from build123d import *

# Parameters (mm, degrees)
SKETCH1_R           = 4
SKETCH1_R_2         = 11
BOSS_EXTRUDE1_DEPTH = 10
BOSS_EXTRUDE2_DEPTH = 20
BOSS_EXTRUDE3_DEPTH = 5
SKETCH6_R           = 11
CUT_EXTRUDE2_DEPTH  = 7
CUT_EXTRUDE3_REACH  = 123.903
SKETCH3_R           = 4
FILLET1_R           = 5


with BuildPart() as part:
    # Sketch1 → Boss-Extrude1 (new body)
    # profile 1 of 4: a face of its own
    with BuildSketch(Plane(origin=(0, 0, 0), x_dir=(1, 0, 0), z_dir=(0, 1, 0))):
        with BuildLine():
            ThreePointArc((-15.53030303, -17.49196326), (-18.965809959, -17.990656132), (-22.023809524, -19.633836312))
            ThreePointArc((-22.023809524, -19.633836312), (-40.737950416, -24.78942672), (-57.5, -15))
            Line((-57.5, -15), (-57.5, 15))
            ThreePointArc((-57.5, 15), (-40.737950416, 24.78942672), (-22.023809524, 19.633836312))
            ThreePointArc((-22.023809524, 19.633836312), (-18.965809959, 17.990656132), (-15.53030303, 17.49196326))
            ThreePointArc((-15.53030303, 17.49196326), (-10.248929974, 16.842723462), (-5.406818182, 14.63628582))
            ThreePointArc((-5.406818182, 14.63628582), (-2.801045952, 13.422385369), (0.042391304, 12.999930884))
            ThreePointArc((0.042391304, 12.999930884), (13, 0), (0.042391304, -12.999930884))
            ThreePointArc((0.042391304, -12.999930884), (-2.801045952, -13.422385369), (-5.406818182, -14.63628582))
            ThreePointArc((-5.406818182, -14.63628582), (-10.248929974, -16.842723462), (-15.53030303, -17.49196326))
        make_face()
        with Locations((-37.5, 0)):
            Circle(SKETCH1_R, mode=Mode.SUBTRACT)
        Circle(SKETCH1_R_2, mode=Mode.SUBTRACT)
        with Locations((-15, 0)):
            Circle(SKETCH1_R, mode=Mode.SUBTRACT)
    # profile 2 of 4: a face of its own
    with BuildSketch(Plane(origin=(0, 0, 0), x_dir=(1, 0, 0), z_dir=(0, 1, 0))):
        with Locations((-37.5, 0)):
            Circle(SKETCH1_R)
    # profile 3 of 4: a face of its own
    with BuildSketch(Plane(origin=(0, 0, 0), x_dir=(1, 0, 0), z_dir=(0, 1, 0))):
        with Locations((-15, 0)):
            Circle(SKETCH1_R)
    # profile 4 of 4: a face of its own
    with BuildSketch(Plane(origin=(0, 0, 0), x_dir=(1, 0, 0), z_dir=(0, 1, 0))):
        Circle(SKETCH1_R_2)
    extrude(amount=BOSS_EXTRUDE1_DEPTH)

    # Sketch1<3> → Boss-Extrude2 (add)
    with BuildSketch(Plane(origin=(0, 0, 0), x_dir=(1, 0, 0), z_dir=(0, 1, 0))):
        with BuildLine():
            Line((-67.5, -18.027756377), (-67.5, 18.027756377))
            ThreePointArc((-67.5, 18.027756377), (-43.803347329, 34.427718665), (-15.833333333, 27.487370837))
            ThreePointArc((-15.833333333, 27.487370837), (-7.534032816, 26.467136868), (0.075, 22.999877717))
            ThreePointArc((0.075, 22.999877717), (23, 0), (0.075, -22.999877717))
            ThreePointArc((0.075, -22.999877717), (-7.534032816, -26.467136868), (-15.833333333, -27.487370837))
            ThreePointArc((-15.833333333, -27.487370837), (-43.803347329, -34.427718665), (-67.5, -18.027756377))
        make_face()
        with BuildLine():
            Line((-57.5, -15), (-57.5, 15))
            ThreePointArc((-57.5, 15), (-40.737950416, 24.78942672), (-22.023809524, 19.633836312))
            ThreePointArc((-22.023809524, 19.633836312), (-18.965809959, 17.990656132), (-15.53030303, 17.49196326))
            ThreePointArc((-15.53030303, 17.49196326), (-10.248929974, 16.842723462), (-5.406818182, 14.63628582))
            ThreePointArc((-5.406818182, 14.63628582), (-2.801045952, 13.422385369), (0.042391304, 12.999930884))
            ThreePointArc((0.042391304, 12.999930884), (13, 0), (0.042391304, -12.999930884))
            ThreePointArc((0.042391304, -12.999930884), (-2.801045952, -13.422385369), (-5.406818182, -14.63628582))
            ThreePointArc((-5.406818182, -14.63628582), (-10.248929974, -16.842723462), (-15.53030303, -17.49196326))
            ThreePointArc((-15.53030303, -17.49196326), (-18.965809959, -17.990656132), (-22.023809524, -19.633836312))
            ThreePointArc((-22.023809524, -19.633836312), (-40.737950416, -24.78942672), (-57.5, -15))
        make_face(mode=Mode.SUBTRACT)
    extrude(amount=BOSS_EXTRUDE2_DEPTH)

    # Sketch2 → Boss-Extrude3 (add)
    with BuildSketch(Plane(origin=(0, 20, 0), x_dir=(1, 0, 0), z_dir=(0, 1, 0))):
        with BuildLine():
            Line((-77.5, -20.615528128), (-77.5, 20.615528128))
            ThreePointArc((-77.5, 20.615528128), (-48.761384661, 43.568121551), (-12.5, 37.416573868))
            ThreePointArc((-12.5, 37.416573868), (-4.462855904, 35.989145507), (3.075, 32.856420605))
            ThreePointArc((3.075, 32.856420605), (33, 0), (3.075, -32.856420605))
            ThreePointArc((3.075, -32.856420605), (-4.462855904, -35.989145507), (-12.5, -37.416573868))
            ThreePointArc((-12.5, -37.416573868), (-48.761384661, -43.568121551), (-77.5, -20.615528128))
        make_face()
        with BuildLine():
            Line((-57.5, -15), (-57.5, 15))
            ThreePointArc((-57.5, 15), (-40.737950416, 24.78942672), (-22.023809524, 19.633836312))
            ThreePointArc((-22.023809524, 19.633836312), (-18.965809959, 17.990656132), (-15.53030303, 17.49196326))
            ThreePointArc((-15.53030303, 17.49196326), (-10.248929974, 16.842723462), (-5.406818182, 14.63628582))
            ThreePointArc((-5.406818182, 14.63628582), (-2.801045952, 13.422385369), (0.042391304, 12.999930884))
            ThreePointArc((0.042391304, 12.999930884), (13, 0), (0.042391304, -12.999930884))
            ThreePointArc((0.042391304, -12.999930884), (-2.801045952, -13.422385369), (-5.406818182, -14.63628582))
            ThreePointArc((-5.406818182, -14.63628582), (-10.248929974, -16.842723462), (-15.53030303, -17.49196326))
            ThreePointArc((-15.53030303, -17.49196326), (-18.965809959, -17.990656132), (-22.023809524, -19.633836312))
            ThreePointArc((-22.023809524, -19.633836312), (-40.737950416, -24.78942672), (-57.5, -15))
        make_face(mode=Mode.SUBTRACT)
    extrude(amount=BOSS_EXTRUDE3_DEPTH)

    # Sketch6 → Cut-Extrude2 (cut)
    with BuildSketch(Plane(origin=(-57.5, 0, 0), x_dir=(0, 0, -1), z_dir=(1, 0, 0))):
        with Locations((0.437281594, 25)):
            Circle(SKETCH6_R)
    extrude(amount=-CUT_EXTRUDE2_DEPTH, mode=Mode.SUBTRACT)

    # Sketch3 → Cut-Extrude3 (cut, up to next)
    with BuildSketch(Plane.ZY.offset(77.5), mode=Mode.PRIVATE) as cut_extrude3_sk1:
        with Locations((0, 25)):
            Circle(SKETCH3_R)
    cut_extrude3_tool1 = extrude(cut_extrude3_sk1.sketch, amount=-CUT_EXTRUDE3_REACH, mode=Mode.PRIVATE) & part.part
    add(cut_extrude3_tool1.solids().sort_by_distance((-77.5, 25, 0))[0], mode=Mode.SUBTRACT)

    # Fillet1
    fillet1_edges = [part.edges().sort_by_distance(p)[0] for p in [
        (-43.803347329, 0, 34.427718665),
        (-7.534032816, 0, 26.467136868),
        (23, 0, 0),
        (-7.534032816, 0, -26.467136868),
        (-43.803347329, 0, -34.427718665),
        (-67.5, 0, 0),
    ]]
    fillet(fillet1_edges, radius=FILLET1_R - 0.0001)  # a hair under: the kernel refuses the full size


solid = part.part
Could you check a few things on this model? Use its own coordinates, in mm. A direction names the side the tool comes from. Give positions to 0.01 mm unless a question says otherwise; leave off trailing zeros. Order: outer loops, then holes, each group sorted by start corner. A loop starts at its lowest first (then second) coordinate and runs counter-clockwise, first axis right, second up. Notation, with made-up numbers: (64.25, 32) -> (88.25, 32) arc R11 ccw to (88.25, 39) -> close; hole circle Ø9 at (-22, -35.5). An arc over 180 degrees is marked (long way). Answer in a Markdown table with one row per item. Add a question column.
Item 1: Imagine slicing it at C-C (x = -70.5). List the corners of the cut face in (y, z) for me, and give its area (3 significant figures).
Item 2: Please list where these lines run through material, in increasing order: probe 1 along Z at (x, y) = (-38, 17.75) (3 decimals); probe 2 along X at (y, z) = (12, -8.5); probe 3 along Y at (x, z) = (22, 7.5).
Item 3: I'm going to push flat-ended pins straight in: P1, Ø10, axis at x = 4.5, y = 17.5, coming from the +Z side; P2, Ø5.5, axis at y = 22, z = -0.5, coming from the +X side; P3, Ø8, axis at x = -10.5, y = 3, coming from the -Z side. Where does each tip first touch, or does it pass through?
Item 4: We'd pull the mould along Z, two halves only. Please class faces 5 (the flat face through (-57.5, 12, 0)), 6 (the cylindrical face through (-49.274, 22.465, -43.432)), 7 (the cylindrical face through (-4.353, 22.465, 35.957)): pulls with the +Z half, pulls with the -Z half, needs draft (parallel to the pull), parting line crosses it, or undercut.
Item 5: Imagine slicing it at A-A (y = 11.75). List the corners of the cut face in (x, z) for me (3 decimals), and give its area (3 significant figures).
Item 6: For faces 1 (the cylindrical face through (-71, 21, 0)), 2 (the cylindrical face through (-43.4, 12.4, 34.5)), 3 (the flat face through (-64.5, 20, 0)), 4 (the cylindrical face through (22.994, 12.395, -0.505)), which set-ups out of +Z, -Z, +X, -X, +Y, -Y let a thin tool reach every point of the face, with its end or its side?
Item 7: Imagine slicing it at D-D (y = 2.75). List the corners of the cut face in (x, z) for me, and give its area (3 significant figures).
Item 8: Imagine slicing it at B-B (z = 0). List the corners of the cut face in (x, y) for me, and give its area (3 significant figures).
Result:
| question | item | result |
|---|---|---|
| 1 | outline | (20, -30.59) -> (25, -30.59) -> (25, -4) arc R4 cw to (25, 4) -> (25, 30.59) -> (20, 30.59) -> close |
| 1 | area | 281 mm2 |
| 2 | probe 1 | -34.996 to -24.995, 24.995 to 34.996 |
| 2 | probe 2 | -67.5 to -57.5, 9.84 to 21.37 |
| 2 | probe 3 | 20 to 25 |
| 3 | P1 | z = 34.29 |
| 3 | P2 | x = 33 |
| 3 | P3 | z = -27.48 |
| 4 | face 5 | undercut |
| 4 | face 6 | pulls with the -Z half |
| 4 | face 7 | pulls with the +Z half |
| 5 | outline | (-67.5, -18.028) arc R35 ccw to (-15.833, -27.487) arc R27.5 ccw to (0.075, -23) arc R23 ccw to (0.075, 23) arc R27.5 ccw to (-15.833, 27.487) arc R35 ccw to (-67.5, 18.028) -> close; hole (-57.5, -15) arc R25 ccw to (-22.024, -19.634) arc R10 cw to (-15.53, -17.492) arc R17.5 ccw to (-5.407, -14.636) arc R10 cw to (0.042, -13) arc R13 ccw to (0.042, 13) arc R10 cw to (-5.407, 14.636) arc R17.5 ccw to (-15.53, 17.492) arc R10 cw to (-22.024, 19.634) arc R25 ccw to (-57.5, 15) -> close |
| 5 | area | 2,290 mm2 |
| 6 | face 1 | -X, +Y |
| 6 | face 2 | +Z, -Y |
| 6 | face 3 | +Y |
| 6 | face 4 | +X, -Y |
| 7 | outline | (-66.97, -17.88) arc R34.47 ccw to (-16.01, -26.95) arc R26.97 ccw to (-0.09, -22.47) arc R22.47 ccw (long way) to (-0.09, 22.47) arc R26.97 ccw to (-16.01, 26.95) arc R34.47 ccw to (-66.97, 17.88) -> close |
| 7 | area | 4,740 mm2 |
| 8 | outline | (-77.5, 20) -> (-67.5, 20) -> (-67.5, 5) arc R5 ccw to (-62.5, 0) -> (18, 0) arc R5 ccw to (23, 5) -> (23, 20) -> (33, 20) -> (33, 25) -> (13, 25) -> (13, 10) -> (-57.5, 10) -> (-57.5, 14.01) -> (-64.5, 14.01) -> (-64.5, 21) -> (-77.5, 21) -> close |
| 8 | area | 1,170 mm2 |
